Check sheet for the drawn part. Datum: minimum x, y, z corner. Units: mm. A direction names the side the tool comes from. Coordinates: 2 decimals unless noted, no trailing zeros. Write each loop counter-clockwise with the first axis right and the second up, starting at its lowest first coordinate (ties: lowest second). Pieces come first, ordered by that corner, then holes. Notation, with made-up numbers: (78.5, -10.5) -> (113.5, -10.5) arc R18 cw to (113.5, 14.5) -> close; hole circle Ø11 at (-16.5, -31.75). An arc over 180 degrees is marked (long way). Answer in a Markdown table with one row per item.
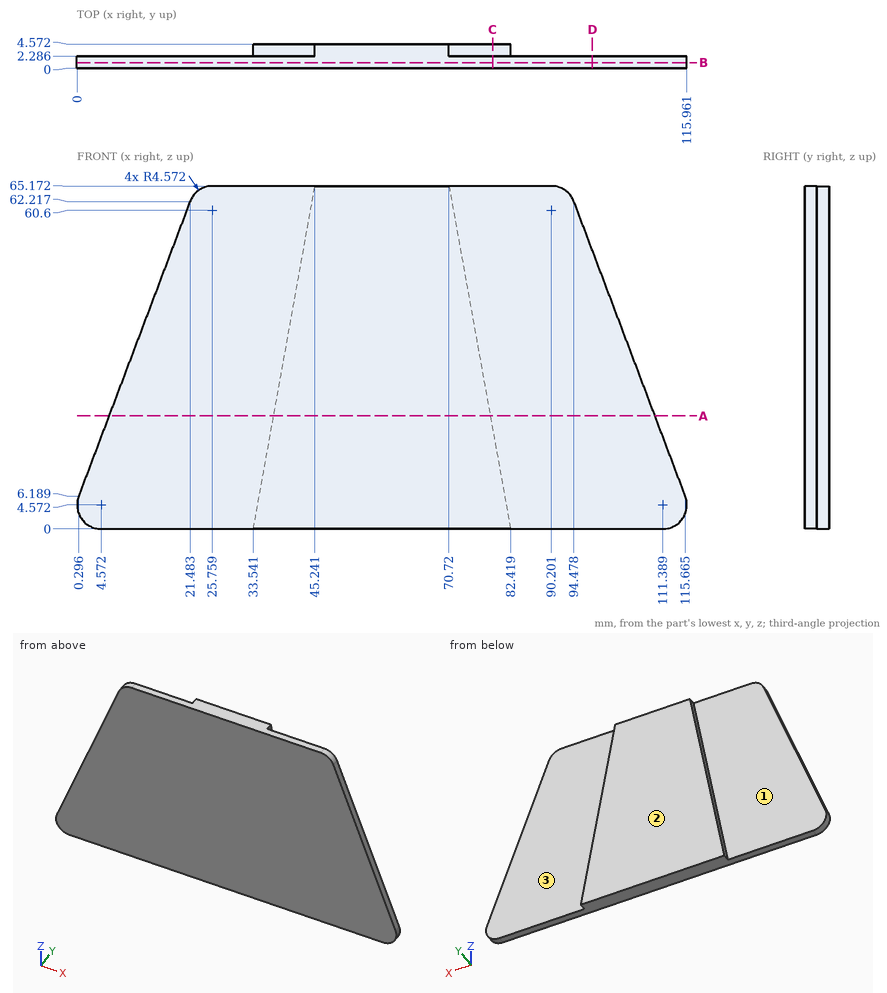
1. Go/stop test with a flat-tipped pin: pin 1 (10 mm diameter, centred on x = 27, z = 16, fed in from +Y). Record where the tip stops, or that it passes through.
Findings below:
| item | result |
|---|---|
| pin 1 | stops at y = 2.29 |
2. Sectioned sample at C-C, the plane x = 79. Record the cut outline in (y, z).
Findings below:
| item | result |
|---|---|
| outline | (0, 0) -> (4.57, 0) -> (4.57, 19.05) -> (2.29, 19.05) -> (2.29, 65.17) -> (0, 65.17) -> close |
3. Sectioned sample at B-B, the plane y = 1.05. Record the cut outline in (x, z) (1 decimal).
Findings below:
| item | result |
|---|---|
| outline | (0.3, 6.2) arc R4.6 ccw to (4.6, 0) -> (111.4, 0) arc R4.6 ccw to (115.7, 6.2) -> (94.5, 62.2) arc R4.6 ccw to (90.2, 65.2) -> (25.8, 65.2) arc R4.6 ccw to (21.5, 62.2) -> close |
4. Sectioned sample at A-A, the plane z = 21.5. Record the cut outline in (x, y) (1 decimal).
Findings below:
| item | result |
|---|---|
| outline | (6.1, 0) -> (109.9, 0) -> (109.9, 2.3) -> (78.6, 2.3) -> (78.6, 4.6) -> (37.4, 4.6) -> (37.4, 2.3) -> (6.1, 2.3) -> close |
5. Access from +Z, -Z, +X, -X, +Y, -Y to the whole of each face (thin tool, end or side, straight path). Record for the marked faces 1, 2 and 3.
Findings below:
| item | result |
|---|---|
| face 1 | +Z, -X, +Y |
| face 2 | +Z, -Z, +X, -X, +Y |
| face 3 | +Z, +X, +Y |
6. Material ranges on probe 1 along Y at (x, z) = (18, 42); probe 2 along X at (y, z) = (3.85, 6.5); probe 3 along X at (y, z) = (2.4, 28), recorded low to high. Write a range as from..to.
Findings below:
| item | result |
|---|---|
| probe 1 | y = 0..2.29 |
| probe 2 | x = 34.71..81.25 |
| probe 3 | x = 38.57..77.39 |
7. Sectioned sample at D-D, the plane x = 98. Record the cut outline in (y, z), and give its area (3 significant figures).
Findings below:
| item | result |
|---|---|
| outline | (0, 0) -> (2.29, 0) -> (2.29, 52.9) -> (0, 52.9) -> close |
| area | 121 mm² |
